Source: CAD feature listing. Evaluate the final solid. Frame: model axes, mm. Face numbers are marked on the shaded views. A direction names the side the tool comes from. Give positions to 0.01 mm unless a question says otherwise; leave off trailing zeros. Loops run counter-clockwise (first coordinate to the right, second up) from the corner with the lowest first, then second, coordinate; pieces in that order, holes last. Notation, with made-up numbers: (32, 38) - (56, 38) arc R19 ccw to (56, 67) - close; hole circle Ø5 at (69, 39). An arc over 180 degrees is marked (long way). Write each question's results on one line, items separated by ' | '. Start each with the question number.
(1) Reachability of the marked faces 4, 5 and 6 from +Z, -Z, +X, -X, +Y, -Y: full face, straight path, thin tool, end or side. Return the list, or none.
(2) Cut plane C-C on x = -5.5. Return the cut outline in (y, z), then the cut area to 3 significant figures.
(3) Pull-direction query (X, two-part tool) for the marked faces 1, 2 and 3; classes: pulls with the +X half, pulls with the -X half, needs draft (parallel to the pull), parting line crosses it, or undercut.
(4) Cut plane B-B on z = 0. Return the cut outline in (x, y), then the cut area to 3 significant figures.
(5) Material intervals for line 1 along Y through (x, z) = (-3, -3.5); line 2 along X through (y, z) = (5.5, -12.5); line 3 along Y through (x, z) = (5.5, -2), sorted ascending. Write a range as [from, to].
(6) Contact query for a flat-ended pin moving along its axis: pin 1 (4 mm diameter, centred on y = 33.5, z = -1, fed in from +X). Output: stop coordinate, or through.
(7) Cut plane A-A on x = 4. Return the cut outline in (y, z), then the cut area to 3 significant figures.
(8) Cut plane D-D on y = 35. Return the cut outline in (x, z), then the cut area to 3 significant figures.
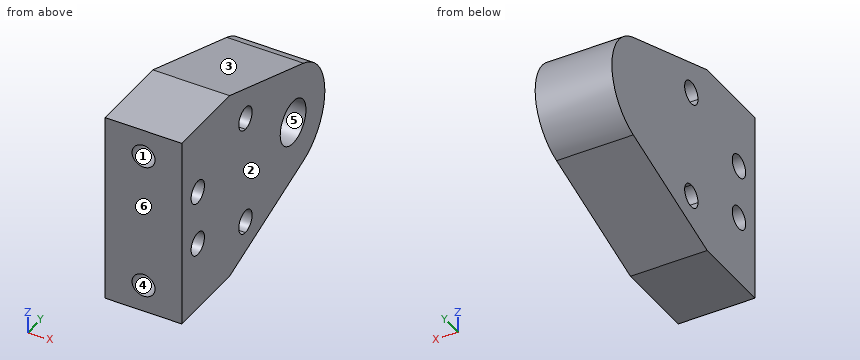
from build123d import *

# Parameters (mm, degrees)
SKETCH_1_W          = 14
SKETCH_1_H          = 35
EXTRUDE_1_DEPTH     = 60
CUT_EXTRUDE_1_DEPTH = 60
SKETCH_3_R          = 2.1
CUT_EXTRUDE_2_DEPTH = 10
SKETCH_4_R          = 4.05
CUT_EXTRUDE_3_DEPTH = 46
CUT_EXTRUDE_4_DEPTH = 100
SKETCH_7_R          = 4.05
EXTRUDE_3_DEPTH     = 2


with BuildPart() as part:
    # 草图1 → 凸台-拉伸1 (new body)
    with BuildSketch(Plane(origin=(0, 0, 0), x_dir=(1, 0, 0), z_dir=(0, 1, 0))):
        Rectangle(SKETCH_1_W, SKETCH_1_H)
    extrude(amount=EXTRUDE_1_DEPTH)

    # 草图2 → 切除-拉伸1 (cut)
    with BuildSketch(Plane(origin=(7, 0, 0), x_dir=(0, 0, -1), z_dir=(1, 0, 0))):
        with BuildLine():
            Line((-17.5, 15), (-9.450519182, 38.269202838))
            ThreePointArc((-9.450519182, 38.269202838), (-5.87e-07, 45), (9.450518798, 38.269203948))
            Line((9.450518798, 38.269203948), (17.5, 15))
            Line((17.5, 15), (17.5, 60))
            Line((17.5, 60), (-17.5, 60))
            Line((-17.5, 60), (-17.5, 15))
        make_face()
    extrude(amount=-CUT_EXTRUDE_1_DEPTH, mode=Mode.SUBTRACT)

    # 草图3 → 切除-拉伸2 (cut)
    with BuildSketch(Plane.XZ):
        with Locations(Location((0, -12.5, 0), (0, 0, 270))):
            Circle(SKETCH_3_R)
        with Locations(Location((0, 12.5, 0), (0, 0, 270))):
            Circle(SKETCH_3_R)
    extrude(amount=-CUT_EXTRUDE_2_DEPTH, mode=Mode.SUBTRACT)

    # 草图4 → 切除-拉伸3 (cut)
    with BuildSketch(Plane(origin=(7, 0, 0), x_dir=(0, 0, -1), z_dir=(1, 0, 0))):
        with Locations((0, 35)):
            Circle(SKETCH_4_R)
    extrude(amount=-CUT_EXTRUDE_3_DEPTH, mode=Mode.SUBTRACT)

    # 草图5 → 切除-拉伸4 (cut)
    with BuildSketch(Plane(origin=(7, 0, 0), x_dir=(0, 0, -1), z_dir=(1, 0, 0))):
        with BuildLine():
            ThreePointArc((-7.9, 20), (-11.48492424, 21.48492424), (-10, 17.9))
            Line((-10, 17.9), (-10, 20))
            Line((-10, 20), (-7.9, 20))
        make_face()
        with BuildLine():
            Line((-10, 20), (-10, 17.9))
            ThreePointArc((-10, 17.9), (-8.51507576, 18.51507576), (-7.9, 20))
            Line((-7.9, 20), (-10, 20))
        make_face()
        with BuildLine():
            ThreePointArc((-7.9, 20), (-11.48492424, 21.48492424), (-10, 17.9))
            Line((-10, 17.9), (-10, 20))
            Line((-10, 20), (-7.9, 20))
        make_face()
        with BuildLine():
            Line((-10, 20), (-10, 17.9))
            ThreePointArc((-10, 17.9), (-8.51507576, 18.51507576), (-7.9, 20))
            Line((-7.9, 20), (-10, 20))
        make_face()
        with BuildLine():
            ThreePointArc((7.9, 20), (8.51507576, 18.51507576), (10, 17.9))
            Line((10, 17.9), (10, 20))
            Line((10, 20), (7.9, 20))
        make_face()
        with BuildLine():
            Line((10, 20), (10, 17.9))
            ThreePointArc((10, 17.9), (11.48492424, 18.51507576), (12.1, 20))
            ThreePointArc((12.1, 20), (10, 22.1), (7.9, 20))
            Line((7.9, 20), (10, 20))
        make_face()
        with BuildLine():
            ThreePointArc((7.9, 20), (8.51507576, 18.51507576), (10, 17.9))
            Line((10, 17.9), (10, 20))
            Line((10, 20), (7.9, 20))
        make_face()
        with BuildLine():
            Line((10, 20), (10, 17.9))
            ThreePointArc((10, 17.9), (11.48492424, 18.51507576), (12.1, 20))
            ThreePointArc((12.1, 20), (10, 22.1), (7.9, 20))
            Line((7.9, 20), (10, 20))
        make_face()
        with BuildLine():
            ThreePointArc((2.9, 5), (5, 2.9), (7.1, 5))
            Line((7.1, 5), (2.9, 5))
        make_face()
        with BuildLine():
            Line((2.9, 5), (7.1, 5))
            ThreePointArc((7.1, 5), (5, 7.1), (2.9, 5))
        make_face()
        with BuildLine():
            ThreePointArc((2.9, 5), (5, 2.9), (7.1, 5))
            Line((7.1, 5), (2.9, 5))
        make_face()
        with BuildLine():
            Line((2.9, 5), (7.1, 5))
            ThreePointArc((7.1, 5), (5, 7.1), (2.9, 5))
        make_face()
        with BuildLine():
            ThreePointArc((-2.9, 5), (-5, 7.1), (-7.1, 5))
            Line((-7.1, 5), (-2.9, 5))
        make_face()
        with BuildLine():
            Line((-2.9, 5), (-7.1, 5))
            ThreePointArc((-7.1, 5), (-5, 2.9), (-2.9, 5))
        make_face()
        with BuildLine():
            ThreePointArc((-2.9, 5), (-5, 7.1), (-7.1, 5))
            Line((-7.1, 5), (-2.9, 5))
        make_face()
        with BuildLine():
            Line((-2.9, 5), (-7.1, 5))
            ThreePointArc((-7.1, 5), (-5, 2.9), (-2.9, 5))
        make_face()
    extrude(amount=-CUT_EXTRUDE_4_DEPTH, mode=Mode.SUBTRACT)


with BuildPart() as body_2:
    # 草图7 → 凸台-拉伸3 (new body)
    with BuildSketch(Plane.ZY.offset(7)):
        with Locations((0, 35)):
            Circle(SKETCH_7_R)
    extrude(amount=-EXTRUDE_3_DEPTH)


with BuildPart() as part_1:
    add(part.part)

    # Combine 1: union body 2
    add(body_2.part)


solid = part_1.part
Ans:
1) face 4: -Y | face 5: +X | face 6: +Z, -Z, +X, -X, -Y
2) outline: (0, -17.5) - (15, -17.5) - (38.27, -9.45) arc R10 ccw to (38.27, 9.45) - (15, 17.5) - (0, 17.5) - close; hole circle Ø4.2 at (5, -5); hole circle Ø4.2 at (5, 5); hole circle Ø4.2 at (20, -10); hole circle Ø4.2 at (20, 10) | area: 1,190 mm^2
3) face 1: undercut | face 2: pulls with the +X half | face 3: needs draft
4) outline: (-7, 0) - (7, 0) - (7, 30.95) - (-5, 30.95) - (-5, 39.05) - (7, 39.05) - (7, 45) - (-7, 45) - close | area: 533 mm^2
5) line 1: [0, 3.53], [6.47, 32.96], [37.04, 44.37] | line 2: [-7, -2.1], [2.1, 7] | line 3: [0, 31.48], [38.52, 44.8]
6) pin 1: x = -5
7) outline: (0, -17.5) - (15, -17.5) - (38.27, -9.45) arc R10 ccw to (38.27, 9.45) - (15, 17.5) - (0, 17.5) - close; hole circle Ø4.2 at (5, -5); hole circle Ø4.2 at (5, 5); hole circle Ø4.2 at (20, -10); hole circle Ø4.2 at (20, 10); hole circle Ø8.1 at (35, 0) | area: 1,140 mm^2
8) outline: (-7, -10.58) - (7, -10.58) - (7, -4.05) - (-5, -4.05) - (-5, 4.05) - (7, 4.05) - (7, 10.58) - (-7, 10.58) - close | area: 199 mm^2
